For this review, take the finished solid that the model builds, in its own axes (mm). A direction names the side the tool comes from. Coordinates: 2 decimals unless noted, no trailing zeros. Order: outer loops, then holes, each group sorted by start corner. A loop starts at its lowest first (then second) coordinate and runs counter-clockwise, first axis right, second up. Notation, with made-up numbers: (84, 78.25) -> (106, 78.25) arc R23 cw to (106, 109.25) -> close; hole circle Ø8 at (-7.75, -35). An arc over 180 degrees is marked (long way). Write item = value, one per line. Start each with the question number.
1) Consider section A-A on z = 0. Give the boundary of the cut face in (x, y), and give its area (3 significant figures).
2) Draft analysis for pull direction Z (two halves, no side actions). For faces 5 (the face through (0, 8.8, -4.4)), 6 (the face through (-0.54, 8.04, -2.44)), 7 (the face through (0, 13, 4)), state which applies: +Z half, -Z half, draft (parallel to the pull), parting line (faces both ways), or undercut.
3) Consider section B-B on x = 2. Give the boundary of the cut face in (y, z), and give its area (3 significant figures).
4) Wall thickness on probe 1 along X at (y, z) = (3.25, 0); probe 2 along Z at (x, y) = (0, 12.5): over which ranges is each line inside the solid? List them lowest first. Write a range as [from, to].
5) Consider section C-C on y = 12. Give the boundary of the cut face in (x, z), and give its area (3 significant figures).
6) Insertion check: pin 1 Ø5 at (y, z) = (10.5, -3) entering from -X; pin 2 Ø0.8 at (x, z) = (-1, 4.5) entering from +Y; pin 3 Ø6 at (x, y) = (-2.5, 14.5) entering from +Z. Each pin has a flat end and moves straight along its axis. Give the tip position at first contact, or say it passes through.
7) Consider section D-D on x = -1.75. Give the boundary of the cut face in (y, z).
8) Machinability: for faces 1 (the face through (0, 8.8, 4.4)), 2 (the face through (-5, 7, 0)), 3 (the face through (0, 13, -4)), 4 (the face through (-5.2, 0, 0.4)), which of the approach directions +Z, -Z, +X, -X, +Y, -Y give a long, thin tool a straight path to every point of the face, cutting with its end or side? Answer none if there is none.
from build123d import *

# Parameters (mm, degrees)
SKETCH_1_R          = 5
SKETCH_1_R_2        = 2.5
EXTRUDE_1_DEPTH     = 17.8
CUT_EXTRUDE_1_DEPTH = 9
SKETCH_4_R          = 2.5
EXTRUDE_2_DEPTH     = 2
FILLET_1_R          = 0.1


with BuildPart() as part:
    # 草图1 → 凸台-拉伸1 (new body)
    with BuildSketch(Plane(origin=(0, 0, 0), x_dir=(1, 0, 0), z_dir=(0, 1, 0))):
        Circle(SKETCH_1_R)
        Circle(SKETCH_1_R_2, mode=Mode.SUBTRACT)
    extrude(amount=EXTRUDE_1_DEPTH)

    # 草图3 → 切除-拉伸1 (cut)
    with BuildSketch(Plane(origin=(0, 17.8, 0), x_dir=(1, 0, 0), z_dir=(0, 1, 0))):
        with BuildLine():
            Line((-3, -4), (3, -4))
            ThreePointArc((3, -4), (0, -5), (-3, -4))
        make_face()
        with BuildLine():
            Line((-3, 4), (3, 4))
            ThreePointArc((3, 4), (0, 5), (-3, 4))
        make_face()
    extrude(amount=-CUT_EXTRUDE_1_DEPTH, mode=Mode.SUBTRACT)

    # 草图4 → 凸台-拉伸2 (add)
    with BuildSketch(Plane.XZ):
        with BuildLine():
            Line((-4.153311931, 5), (4.153311931, 5))
            ThreePointArc((4.153311931, 5), (6.5, 0), (4.153311931, -5))
            Line((4.153311931, -5), (-4.153311931, -5))
            ThreePointArc((-4.153311931, -5), (-6.5, 0), (-4.153311931, 5))
        make_face()
        Circle(SKETCH_4_R, mode=Mode.SUBTRACT)
    extrude(amount=EXTRUDE_2_DEPTH)

    # 圆角1
    fillet_1_edges = [part.edges().sort_by_distance(p)[0] for p in [
        (0, 17.8, 4),
        (-5, 17.8, 0),
        (0, 17.8, -4),
        (4.472135955, 17.8, 2.236067977),
    ]]
    fillet(fillet_1_edges, radius=FILLET_1_R)


solid = part.part
Answer sheet:
q1.outline = (-6.5, -2) -> (-2.5, -2) -> (-2.5, 17.8) -> (-4.9, 17.8) arc R0.1 ccw to (-5, 17.7) -> (-5, 0) -> (-6.5, 0) -> close; (2.5, -2) -> (6.5, -2) -> (6.5, 0) -> (5, 0) -> (5, 17.7) arc R0.1 ccw to (4.9, 17.8) -> (2.5, 17.8) -> close
q1.area = 105 mm2
q2.face_5 = draft
q2.face_6 = undercut
q2.face_7 = +Z half
q3.outline = (-2, -5) -> (0, -5) -> (0, -4.58) -> (8.8, -4.58) -> (8.8, -4) -> (17.7, -4) arc R0.1 ccw to (17.8, -3.9) -> (17.8, -1.5) -> (-2, -1.5) -> close; (-2, 1.5) -> (17.8, 1.5) -> (17.8, 3.9) arc R0.1 ccw to (17.7, 4) -> (8.8, 4) -> (8.8, 4.58) -> (0, 4.58) -> (0, 5) -> (-2, 5) -> close
q3.area = 113 mm2
q4.probe_1 = [-5, -2.5], [2.5, 5]
q4.probe_2 = [-4, -2.5], [2.5, 4]
q5.outline = (-3, -4) -> (3, -4) arc R5 ccw to (3, 4) -> (-3, 4) arc R5 ccw to start; hole circle Ø5 at (0, 0)
q5.area = 50.7 mm2
q6.pin_1 = -4.97
q6.pin_2 = 8.8
q6.pin_3 = 4
q7.outline = (-2, -5) -> (0, -5) -> (0, -4.68) -> (8.8, -4.68) -> (8.8, -4) -> (17.7, -4) arc R0.1 ccw to (17.8, -3.9) -> (17.8, -1.79) -> (-2, -1.79) -> close; (-2, 1.79) -> (17.8, 1.79) -> (17.8, 3.9) arc R0.1 ccw to (17.7, 4) -> (8.8, 4) -> (8.8, 4.68) -> (0, 4.68) -> (0, 5) -> (-2, 5) -> close
q8.face_1 = +Z, +X, -X, +Y
q8.face_2 = +Y
q8.face_3 = -Z, +X, -X, +Y
q8.face_4 = -X, +Y
